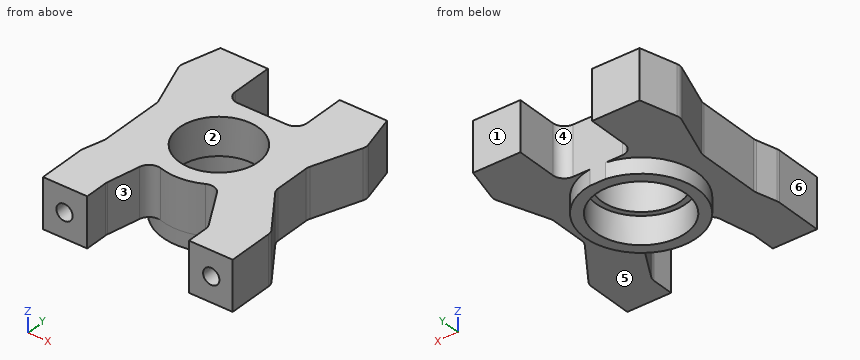
from build123d import *

# Parameters (mm, degrees)
SKETCH1_R           = 7.112
BOSS_EXTRUDE1_DEPTH = 8.89
SKETCH2_R           = 8.1026
BOSS_EXTRUDE2_DEPTH = 2.794
CUT_EXTRUDE1_START  = -2.1844
SKETCH4_R           = 8.1026
CUT_EXTRUDE1_DEPTH  = 2.1844
SKETCH5_R           = 1.4605
CUT_EXTRUDE2_DEPTH  = 7.62


with BuildPart() as part:
    # Sketch1 → Boss-Extrude1 (new body)
    with BuildSketch(Plane.XY):
        with BuildLine():
            Line((4.4196, 9.970322522), (-4.4196, 9.970322522))
            ThreePointArc((-4.4196, 9.970322522), (-5.856440979, 10.565481542), (-6.4516, 12.002322522))
            Line((-6.4516, 12.002322522), (-6.4516, 19.469922522))
            Line((-6.4516, 19.469922522), (-14.9606, 19.469922522))
            Line((-14.9606, 19.469922522), (-16.647754284, 13.056434928))
            ThreePointArc((-16.647754284, 13.056434928), (-16.712590479, 12.448835423), (-16.593859144, 11.849432587))
            Line((-16.593859144, 11.849432587), (-13.582754018, 3.50945712))
            ThreePointArc((-13.582754018, 3.50945712), (-13.492416148, 3.169677348), (-13.462, 2.819411617))
            Line((-13.462, 2.819411617), (-13.462, 0))
            Line((-13.462, 0), (-13.462, -8.647780438))
            ThreePointArc((-13.462, -8.647780438), (-13.478784036, -8.908411634), (-13.528858878, -9.164737275))
            Line((-13.528858878, -9.164737275), (-14.461941122, -12.711722544))
            ThreePointArc((-14.461941122, -12.711722544), (-14.512015964, -12.968048185), (-14.5288, -13.228679381))
            Line((-14.5288, -13.228679381), (-14.5288, -21.805077478))
            Line((-14.5288, -21.805077478), (-6.5786, -21.805077478))
            Line((-6.5786, -21.805077478), (-6.5786, -17.586954898))
            ThreePointArc((-6.5786, -17.586954898), (-6.568684578, -17.386460615), (-6.539035081, -17.187923011))
            Line((-6.539035081, -17.187923011), (-5.363383159, -11.317690055))
            ThreePointArc((-5.363383159, -11.317690055), (-4.426978503, -9.980685151), (-2.809123398, -9.763934951))
            ThreePointArc((-2.809123398, -9.763934951), (0.991075795, -10.11154631), (4.651460928, -9.032691251))
            ThreePointArc((4.651460928, -9.032691251), (6.155731201, -8.889980119), (7.342613103, -9.82513084))
            Line((7.342613103, -9.82513084), (11.42555999, -16.91467556))
            ThreePointArc((11.42555999, -16.91467556), (11.62774502, -17.403914002), (11.6967, -17.928774222))
            Line((11.6967, -17.928774222), (11.6967, -21.805077478))
            Line((11.6967, -21.805077478), (19.558, -21.805077478))
            Line((19.558, -21.805077478), (19.558, -13.603952816))
            ThreePointArc((19.558, -13.603952816), (19.464666148, -12.995185564), (19.193238615, -12.442342123))
            Line((19.193238615, -12.442342123), (13.826761385, -4.739935355))
            ThreePointArc((13.826761385, -4.739935355), (13.555333852, -4.187091915), (13.462, -3.578324662))
            Line((13.462, -3.578324662), (13.462, 0))
            Line((13.462, 0), (13.462, 2.819411617))
            ThreePointArc((13.462, 2.819411617), (13.492416148, 3.169677348), (13.582754018, 3.50945712))
            Line((13.582754018, 3.50945712), (16.593859144, 11.849432587))
            ThreePointArc((16.593859144, 11.849432587), (16.712590479, 12.448835423), (16.647754284, 13.056434928))
            Line((16.647754284, 13.056434928), (14.9606, 19.469922522))
            Line((14.9606, 19.469922522), (6.4516, 19.469922522))
            Line((6.4516, 19.469922522), (6.4516, 12.002322522))
            ThreePointArc((6.4516, 12.002322522), (5.856440979, 10.565481542), (4.4196, 9.970322522))
        make_face()
        Circle(SKETCH1_R, mode=Mode.SUBTRACT)
    extrude(amount=BOSS_EXTRUDE1_DEPTH)

    # Sketch2 → Boss-Extrude2 (add)
    with BuildSketch(Plane(origin=(0, 0, 0), x_dir=(-1, 0, 0), z_dir=(0, 0, -1))):
        with BuildLine():
            Line((-1.42116995, 9.970322522), (1.42116995, 9.970322522))
            ThreePointArc((1.42116995, 9.970322522), (0, -10.0711), (-1.42116995, 9.970322522))
        make_face()
        Circle(SKETCH2_R, mode=Mode.SUBTRACT)
    extrude(amount=BOSS_EXTRUDE2_DEPTH)

    # Sketch4 → Cut-Extrude1 (cut)
    with BuildSketch(Plane(origin=(0, 0, 0), x_dir=(-1, 0, 0), z_dir=(0, 0, -1)).offset(CUT_EXTRUDE1_START)):
        Circle(SKETCH4_R)
    extrude(amount=CUT_EXTRUDE1_DEPTH, mode=Mode.SUBTRACT)

    # Sketch5 → Cut-Extrude2 (cut)
    with BuildSketch(Plane.XZ.offset(21.805077478)):
        with Locations(Location((-10.668, 4.445, 0), (0, 0, 270))):
            Circle(SKETCH5_R)
        with Locations(Location((15.6972, 4.445, 0), (0, 0, 270))):
            Circle(SKETCH5_R)
    extrude(amount=-CUT_EXTRUDE2_DEPTH, mode=Mode.SUBTRACT)


solid = part.part
CAD build for the part. Positions are in the model's coordinates, mm. Face numbers are marked on the shaded views. A direction names the side the tool comes from. Round coordinates to 2 decimals unless told otherwise and drop trailing zeros. Loops run counter-clockwise (first coordinate to the right, second up) from the corner with the lowest first, then second, coordinate; pieces in that order, holes last.
(1) Wall check: line 1 along Y through (x, z) = (0, 5); line 2 along Y through (x, z) = (0, 0.8); line 3 along X through (y, z) = (0, 5.75). Give the ranges that are in metal, low to high.
(2) Two-plate mould, pull along Y, no slides. Class the marked faces 1, 2 and 3: +Y half, -Y half, draft (parallel to the pull), parting line (faces both ways), or undercut.
(3) Cut at C-C (y = 0). Give the cut face in (x, z).
(4) Cut at A-A (x = 0). Give the cut face in (y, z), plus the area to 3 significant figures.
(5) Cut at B-B (y = -15). Give the cut face in (x, z) (1 decimal).
(6) Which spindle directions (+Z, -Z, +X, -X, +Y, -Y) get a long thin tool onto all of the face, cutting with end or side? Do the marked faces 4, 5 and 6. Say none if no direction does.
(7) Cut at D-D (y = 5). Give the cut face in (x, z).
(8) Drop flat-ended pins along their axis: pin 1 (3.5 mm diameter, centred on y = 14, z = 5, fed in from +X); pin 2 (1.5 mm diameter, centred on y = -8, z = 5.5, fed in from -X); pin 3 (1.5 mm diameter, centred on x = 6, y = 13.5, fed in from -Z); pin 4 (9.5 mm diameter, centred on x = 0, y = 0, fed in from -Z). Give the stop position or say it passes through.
Findings below:
1. line 1: y = -10.16 to -7.11, 7.11 to 9.97
1. line 2: y = -10.16 to -8.1, 8.1 to 9.97
1. line 3: x = -13.46 to -7.11, 7.11 to 13.46
2. face 1: +Y half
2. face 2: undercut
2. face 3: -Y half
3. outline: (-13.46, 0) - (-10.07, 0) - (-10.07, -2.79) - (-8.1, -2.79) - (-8.1, 2.18) - (-7.11, 2.18) - (-7.11, 8.89) - (-13.46, 8.89) - close; (7.11, 2.18) - (8.1, 2.18) - (8.1, -2.79) - (10.07, -2.79) - (10.07, 0) - (13.46, 0) - (13.46, 8.89) - (7.11, 8.89) - close
4. outline: (-10.16, 0) - (-10.07, 0) - (-10.07, -2.79) - (-8.1, -2.79) - (-8.1, 2.18) - (-7.11, 2.18) - (-7.11, 8.89) - (-10.16, 8.89) - close; (7.11, 2.18) - (8.1, 2.18) - (8.1, -2.79) - (9.97, -2.79) - (9.97, 8.89) - (7.11, 8.89) - close
4. area: 58.9 mm2
5. outline: (-14.5, 0) - (-6.1, 0) - (-6.1, 8.9) - (-14.5, 8.9) - close; (10.3, 0) - (19.6, 0) - (19.6, 8.9) - (10.3, 8.9) - close; hole circle Ø2.9 at (-10.7, 4.4); hole circle Ø2.9 at (15.7, 4.4)
6. face 4: +Z, -Z, +Y
6. face 5: -Z
6. face 6: +Z, -Z, -X, -Y
7. outline: (-14.12, 0) - (-8.74, 0) - (-8.74, -2.79) - (-6.38, -2.79) - (-6.38, 2.18) - (-5.06, 2.18) - (-5.06, 8.89) - (-14.12, 8.89) - close; (5.06, 2.18) - (6.38, 2.18) - (6.38, -2.79) - (8.74, -2.79) - (8.74, 0) - (14.12, 0) - (14.12, 8.89) - (5.06, 8.89) - close
8. pin 1: stops at x = 16.71
8. pin 2: stops at x = -13.46
8. pin 3: stops at z = 0
8. pin 4: passes through
